```python
from build123d import *

# Parameters (mm, degrees)
F0_R     = 1.75
F0_R_2   = 4.5
F1_DEPTH = 2
F2_R     = 5


with BuildPart() as f1:
    # F0 (on Top) → F1 (new body)
    with BuildSketch(Plane.XY):
        with BuildLine():
            Line((20, 30), (-20, 30))
            Line((-20, 30), (-20, 22))
            ThreePointArc((-20, 22), (-13.8300253787, 0), (-20, -22))
            Line((-20, -22), (-20, -30))
            Line((-20, -30), (20, -30))
            Line((20, -30), (20, -22))
            ThreePointArc((20, -22), (13.8300253787, 0), (20, 22))
            Line((20, 22), (20, 30))
        make_face()
        with Locations((-16, -26)):
            Circle(F0_R, mode=Mode.SUBTRACT)
        with Locations((-9, -9)):
            Circle(F0_R, mode=Mode.SUBTRACT)
        with Locations((-6.4855394704, -3.7666666667)):
            Circle(F0_R, mode=Mode.SUBTRACT)
        Polygon((10, -22.4003139883), (0, -22.4003139883), (-10, -22.4003139883), (0, -11.7255505174), align=None, mode=Mode.SUBTRACT)
        with Locations((16, -26)):
            Circle(F0_R, mode=Mode.SUBTRACT)
        with Locations((9, -9)):
            Circle(F0_R, mode=Mode.SUBTRACT)
        with Locations((6.4855394704, -3.7666666667)):
            Circle(F0_R, mode=Mode.SUBTRACT)
        with BuildLine():
            ThreePointArc((-10.4007968114, 7.9510632559), (-10.1861204729, 10.2867082901), (-7.840755933, 10.310974139))
            ThreePointArc((-7.840755933, 10.310974139), (-7.7595664935, 10.2344329532), (-7.6834199086, 10.1528733074))
            Line((-7.6834199086, 10.1528733074), (-4.9243436791, 7.3803852648))
            ThreePointArc((-4.9243436791, 7.3803852648), (-4.4275976085, 6.7681475895), (-4.25, 6))
            ThreePointArc((-4.25, 6), (-5.1630952479, 4.4630906221), (-6.9495319267, 4.5300037006))
            ThreePointArc((-6.9495319267, 4.5300037006), (-7.2319861689, 4.7571363391), (-7.4615928772, 5.0375831146))
            Line((-7.4615928772, 5.0375831146), (-10.0365828557, 7.5900368858))
            ThreePointArc((-10.0365828557, 7.5900368858), (-10.2319861689, 7.7571363391), (-10.4007968114, 7.9510632559))
        make_face(mode=Mode.SUBTRACT)
        with Locations((-16, 26)):
            Circle(F0_R, mode=Mode.SUBTRACT)
        Circle(F0_R_2, mode=Mode.SUBTRACT)
        with Locations((0, 7.5)):
            Circle(F0_R, mode=Mode.SUBTRACT)
        with BuildLine():
            ThreePointArc((7.840755933, 10.310974139), (9.7189655356, 10.5954900685), (10.75, 9))
            ThreePointArc((10.75, 9), (10.6604057365, 8.4472317031), (10.4007968114, 7.9510632559))
            ThreePointArc((10.4007968114, 7.9510632559), (10.2319861689, 7.7571363391), (10.0365828557, 7.5900368858))
            Line((10.0365828557, 7.5900368858), (7.4615928772, 5.0375831146))
            ThreePointArc((7.4615928772, 5.0375831146), (7.2319861689, 4.7571363391), (6.9495319267, 4.5300037006))
            ThreePointArc((6.9495319267, 4.5300037006), (4.5734147043, 4.9864150781), (4.9243436791, 7.3803852648))
            Line((4.9243436791, 7.3803852648), (7.6834199086, 10.1528733074))
            ThreePointArc((7.6834199086, 10.1528733074), (7.7595664935, 10.2344329532), (7.840755933, 10.310974139))
        make_face(mode=Mode.SUBTRACT)
        Polygon((0, 22.4003139883), (10, 22.4003139883), (0, 11.7255505174), (-10, 22.4003139883), align=None, mode=Mode.SUBTRACT)
        with Locations((16, 26)):
            Circle(F0_R, mode=Mode.SUBTRACT)
    extrude(amount=F1_DEPTH)

    # F2
    f2_edges = [f1.edges().sort_by_distance(p)[0] for p in [
        (-20, 30, 1),
        (-20, -30, 1),
        (20, -30, 1),
        (20, 30, 1),
        (20, -22, 1),
        (-20, -22, 1),
        (-20, 22, 1),
    ]]
    fillet(f2_edges, radius=F2_R)


solid = f1.part
```
Verification items for the finished model (mm, model axes). A direction names the side the tool comes from. Give positions to 0.01 mm unless a question says otherwise; leave off trailing zeros. Loops run counter-clockwise (first coordinate to the right, second up) from the corner with the lowest first, then second, coordinate; pieces in that order, holes last. Notation, with made-up numbers: M -35.75,-11.5 L -14.75,-11.5 A20 cw -14.75,26.5 Z; hole C 86.5,-14 d2. An arc over 180 degrees is marked long. Return JSON: item names as keys, results as strings.
1) Gauge pin test, flat ends, axial feed: P1, Ø5.5, axis at x = 6.49, y = -3.77, coming from the -Z side; P2, Ø2, axis at x = -9, y = -9, coming from the +Z side. Record the tip position at first contact, or that the pin passes through.
Findings:
{"P1": "stops at z = 0", "P2": "passes through"}
2) Section check D-D, the plane x = -16. Enter the section's corners in (y, z), and give its area (3 significant figures).
Findings:
{"outline": "M -29.9,0 L -27.75,0 L -27.75,2 L -29.9,2 Z; M -24.25,0 L -13.38,0 L -13.38,2 L -24.25,2 Z; M 13.38,0 L 24.25,0 L 24.25,2 L 13.38,2 Z; M 27.75,0 L 29.9,0 L 29.9,2 L 27.75,2 Z", "area": "52.1 mm2"}
3) Tool access check on faces 1 (the flat face through (0, -22.4, 1)), 2 (the flat face through (20, 23, 1)). Record the directions out of +Z, -Z, +X, -X, +Y, -Y that give a thin tool (end or side, any length) a straight path to the whole face; none if there is none.
Findings:
{"face 1": "+Z, -Z", "face 2": "+Z, -Z, +X, +Y, -Y"}
4) Section check B-B, the plane x = 9. Enter the section's corners in (y, z), and give its area (3 significant figures).
Findings:
{"outline": "M -30,0 L -22.4,0 L -22.4,2 L -30,2 Z; M -21.33,0 L -10.75,0 L -10.75,2 L -21.33,2 Z; M -7.25,0 L 6.56,0 L 6.56,2 L -7.25,2 Z; M 10.75,0 L 21.33,0 L 21.33,2 L 10.75,2 Z; M 22.4,0 L 30,0 L 30,2 L 22.4,2 Z", "area": "100 mm2"}
5) Mould release check, pull along X, two halves, no side actions. Record for faces 3 (the cylindrical face through (18, 29, 1)), 4 (the flat face through (0, 30, 1)), 5 (the flat face through (8.767, 6.332, 0.986)), 6 (the cylindrical face through (-13.83, 0.31, 0.99)): released by +X, released by -X, zero draft, split by the parting line, or undercut.
Findings:
{"face 3": "released by +X", "face 4": "zero draft", "face 5": "undercut", "face 6": "released by -X"}
6) Section check A-A, the plane y = 0. Enter the section's corners in (x, z), and give its area (3 significant figures).
Findings:
{"outline": "M -13.83,0 L -4.5,0 L -4.5,2 L -13.83,2 Z; M 4.5,0 L 13.83,0 L 13.83,2 L 4.5,2 Z", "area": "37.3 mm2"}
7) Section check C-C, the plane y = -9. Enter the section's corners in (x, z).
Findings:
{"outline": "M -14.8,0 L -10.75,0 L -10.75,2 L -14.8,2 Z; M -7.25,0 L 7.25,0 L 7.25,2 L -7.25,2 Z; M 10.75,0 L 14.8,0 L 14.8,2 L 10.75,2 Z"}
8) Material ranges on L1, parallel to X at y = 5, z = 1.2; L2, parallel to Y at x = 9, z = 1.65; L3, parallel to Y at x = 2, z = 0.25, recorded low to high. Write a range as [from, to].
Findings:
{"L1": "x = [-14.13, -7.44], [-4.56, 4.56], [7.44, 14.13]", "L2": "y = [-30, -22.4], [-21.33, -10.75], [-7.25, 6.56], [10.75, 21.33], [22.4, 30]", "L3": "y = [-30, -22.4], [-13.86, -4.03], [4.03, 13.86], [22.4, 30]"}
